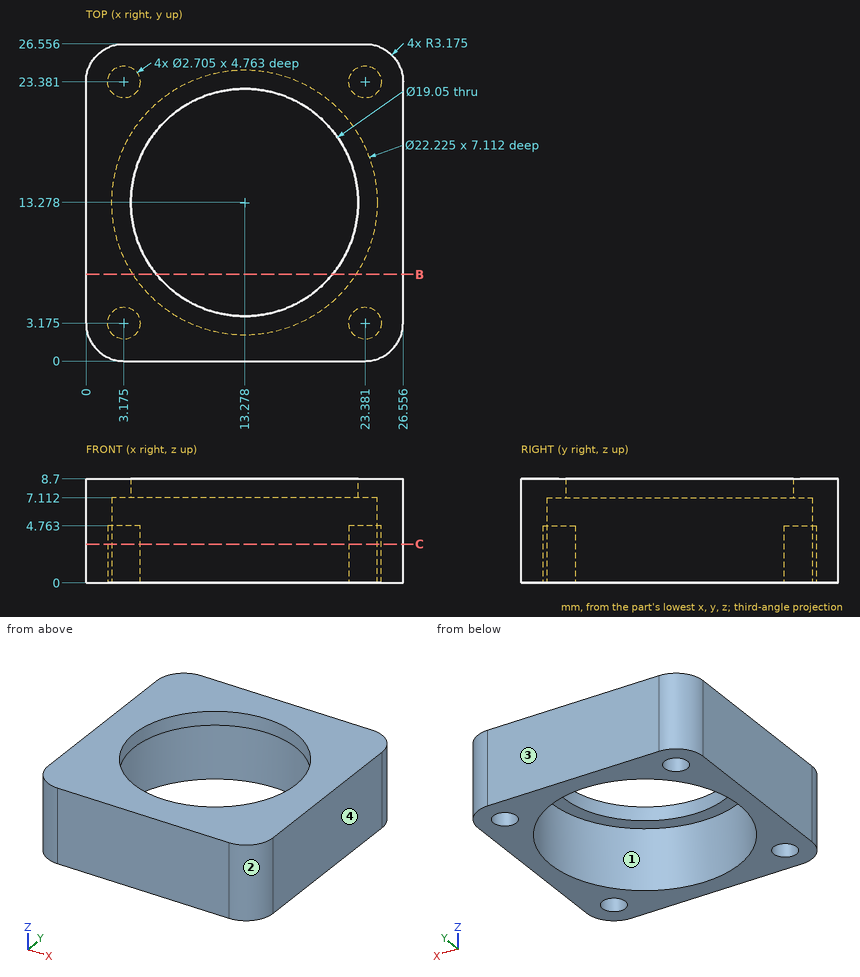
Can you work these out from the drawing? Everything is in mm from the part's minimum corner. Coordinates: 2 decimals unless noted, no trailing zeros. Loops run counter-clockwise (first coordinate to the right, second up) from the corner with the lowest first, then second, coordinate; pieces in that order, holes last.
1. If we mould it in two halves opening along Y, with no side actions, what happens to the marked faces 1, 2, 3 and 4? For each: pulls with the +Y half, pulls with the -Y half, needs draft (parallel to the pull), parting line crosses it, or undercut.
2. Imagine slicing it at C-C, the plane z = 3.25. Count the separate pieces of the cut face and the enclosed holes in it.
3. For P1, Ø0.8, axis at x = 23, y = 23.5, coming from the -Z side; P2, Ø4, axis at x = 21, y = 15, coming from the -Z side, each with a flat end and sliding along its axis, tell me the tip position at first contact or that it passes through.
4. I need wall thicknesses on L1, parallel to Y at x = 22.25, z = 3 (1 decimal); L2, parallel to X at y = 13, z = 3 (1 decimal); L3, parallel to Y at x = 15.75, z = 7.5 (1 decimal). Which ranges of each line are inside material? Lowest first, please.
5. Imagine slicing it at B-B, the plane y = 7.25. Please give me the cut outline in (x, z) (1 decimal).
Taken from the geometry:
1. face 1: undercut
1. face 2: pulls with the -Y half
1. face 3: pulls with the +Y half
1. face 4: needs draft
2. separate pieces: 1
2. enclosed holes: 5
3. P1: stops at z = 4.76
3. P2: stops at z = 7.11
4. L1: y = 0 to 2.4, 3.9 to 6.7, 19.8 to 22.6, 24.1 to 26.6
4. L2: x = 0 to 2.2, 24.4 to 26.6
4. L3: y = 0 to 4.1, 22.5 to 26.6
5. outline: (0, 0) - (3.9, 0) - (3.9, 7.1) - (5.9, 7.1) - (5.9, 8.7) - (0, 8.7) - close; (20.7, 7.1) - (22.6, 7.1) - (22.6, 0) - (26.6, 0) - (26.6, 8.7) - (20.7, 8.7) - close
